Work out the finished part from the listing and answer in its coordinate system (mm). Round coordinates to 2 decimals unless told otherwise and drop trailing zeros. Loops run counter-clockwise (first coordinate to the right, second up) from the corner with the lowest first, then second, coordinate; pieces in that order, holes last.
Autodesk Inventor part; units mm, degrees
ref_plane "Work Plane1" through (0, 58, 0) normal (-1, 0, 0) x (0, 0, 1)
ref_plane "Work Plane2" through (-125, 58, 18) normal (1, 0, 0) x (0, 0, -1)
ref_plane "YZ Plane" through (0, 0, 0) normal (1, 0, 0) x (0, 1, 0)
sketch "Sketch1" plane through (0, 0, 0) normal (0, 0, 1) x (1, 0, 0)
  line L0 (-375, 40) -> (375, 40)
  line L1 (375, 40) -> (375, -40)
  line L2 (375, -40) -> (-375, -40)
  line L3 (-375, -40) -> (-375, 40)
  point P0 (0, 0)
  point P1 (375, 0)
  point P2 (0, 40)
  dimension "d0" = 750
  dimension "d1" = 80
extrude "Extrusion1" add sketch "Sketch1" along normal blind 18
sketch "Sketch2" plane through (0, 0, 18) normal (0, 0, 1) x (1, 0, 0)
  line L0 (375, 40) -> (-375, 40)
  line L1 (-375, 40) -> (-375, -40)
  line L2 (-375, -40) -> (375, -40)
  line L3 (375, -40) -> (375, 40)
  line L4 (-375, 58) -> (-316, 58)
  line L5 (-316, 58) -> (-316, 40)
  line L6 (-316, 40) -> (-375, 40)
  line L7 (-375, 40) -> (-375, 58)
  point P0 (0, 0)
  point P1 (-345.5, 40)
  point P2 (0, 40)
  point P3 (-375, 49)
  point P4 (-375, 0)
  dimension "d4" = 18
  dimension "d5" = 59
extrude "Extrusion2" add sketch "Sketch2" against normal blind 18 contours L0 L7 L4 L5
sketch "Sketch3" plane through (0, 0, 18) normal (0, 0, 1) x (1, 0, 0)
  line L0 (-175, 58) -> (-75, 58)
  line L1 (-75, 58) -> (-75, 40)
  line L2 (-75, 40) -> (-175, 40)
  line L3 (-175, 40) -> (-175, 58)
  line L4 (375, 40) -> (-316, 40)
  line L5 (-316, 58) -> (-316, 40)
  line L6 (-375, 58) -> (-316, 58)
  line L7 (-375, -40) -> (-375, 58)
  line L8 (-375, -40) -> (375, -40)
  line L9 (375, -40) -> (375, 40)
  point P0 (0, 0)
  point P1 (-125, 40)
  point P2 (29.5, 40)
  dimension "d8" = 100
  dimension "d9" = 18
  dimension "d10" = 250
extrude "Extrusion3" add sketch "Sketch3" against normal blind 18 contours L0 L1 L2 L3
sketch "Sketch4" plane through (0, 0, 18) normal (0, 0, 1) x (1, 0, 0)
  line L0 (375, 40) -> (-75, 40)
  line L1 (-75, 58) -> (-75, 40)
  line L2 (-175, 58) -> (-75, 58)
  line L3 (-175, 40) -> (-175, 58)
  line L4 (-175, 40) -> (-316, 40)
  line L5 (-316, 58) -> (-316, 40)
  line L6 (-375, 58) -> (-316, 58)
  line L7 (-375, -40) -> (-375, 58)
  line L8 (-375, -40) -> (375, -40)
  line L9 (375, -40) -> (375, 40)
  line L10 (-375, -40) -> (-357, -40)
  line L11 (-357, -40) -> (-357, 9)
  line L12 (-357, 9) -> (-375, 9)
  line L13 (-375, 9) -> (-375, -40)
  point P0 (0, 0)
  point P1 (-366, -40)
  point P2 (0, -40)
  point P3 (-375, -15.5)
  point P4 (-375, 9)
  dimension "d13" = 18
  dimension "d14" = 49
extrude "Extrusion4" cut sketch "Sketch4" against normal blind 18 contours L8 L7 L12 L11
sketch "Sketch5" plane through (0, 0, 18) normal (0, 0, 1) x (1, 0, 0)
  line L0 (-134, 58) -> (-116, 58)
  line L1 (-116, 58) -> (-116, 9)
  line L2 (-116, 9) -> (-134, 9)
  line L3 (-134, 9) -> (-134, 58)
  line L4 (-375, 9) -> (-357, 9)
  line L5 (-357, 9) -> (-357, -40)
  line L6 (-357, -40) -> (375, -40)
  line L7 (375, -40) -> (375, 40)
  line L8 (375, 40) -> (-75, 40)
  line L9 (-75, 58) -> (-75, 40)
  line L10 (-175, 58) -> (-75, 58)
  line L11 (-175, 40) -> (-175, 58)
  line L12 (-175, 40) -> (-316, 40)
  line L13 (-316, 58) -> (-316, 40)
  line L14 (-375, 58) -> (-316, 58)
  line L15 (-375, 9) -> (-375, 58)
  line L16 (-175, 58) -> (-75, 58)
  point P0 (0, 0)
  point P1 (-125, 58)
  point P2 (-125, 58)
  point P3 (-125, 58)
  dimension "d17" = 18
  dimension "d18" = 49
extrude "Extrusion5" cut sketch "Sketch5" against normal blind 18 contours L0 L1 L2 L3
ref_plane "Work Plane1" through (0, 58, 0) normal (-1, 0, 0) x (0, 0, 1)
mirror "Mirror1" about plane through (0, 58, 0) normal (-1, 0, 0) of "Extrusion5", "Extrusion4", "Extrusion3", "Extrusion2"
sketch "Sketch6" plane through (0, 0, 18) normal (0, 0, 1) x (1, 0, 0)
  line L0 (357, 9) -> (375, 9)
  line L1 (375, 9) -> (375, 58)
  line L2 (375, 58) -> (316, 58)
  line L3 (316, 58) -> (316, 40)
  line L4 (316, 40) -> (175, 40)
  line L5 (175, 40) -> (175, 58)
  line L6 (175, 58) -> (134, 58)
  line L7 (134, 58) -> (134, 9)
  line L8 (134, 9) -> (116, 9)
  line L9 (116, 9) -> (116, 58)
  line L10 (116, 58) -> (75, 58)
  line L11 (75, 58) -> (75, 40)
  line L12 (75, 40) -> (-75, 40)
  line L13 (-75, 58) -> (-75, 40)
  line L14 (-116, 58) -> (-75, 58)
  line L15 (-116, 58) -> (-116, 9)
  line L16 (-116, 9) -> (-134, 9)
  line L17 (-134, 9) -> (-134, 58)
  line L18 (-175, 58) -> (-134, 58)
  line L19 (-175, 40) -> (-175, 58)
  line L20 (-175, 40) -> (-316, 40)
  line L21 (-316, 58) -> (-316, 40)
  line L22 (-375, 58) -> (-316, 58)
  line L23 (-375, 9) -> (-375, 58)
  line L24 (-375, 9) -> (-357, 9)
  line L25 (-357, 9) -> (-357, -40)
  line L26 (-357, -40) -> (357, -40)
  line L27 (357, -40) -> (357, 9)
  point P0 (0, 0)
  point P1 (-357, 5.825)
  point P2 (-312.825, 40)
  dimension "d21" = 3.175
  dimension "d22" = 3.175
hole "Hole1" at (-357, 5.825, 18) at (-312.825, 40, 18) direction (0, 0, -1) diameter 6.35 end through all
mirror "Mirror2" about plane through (0, 58, 0) normal (-1, 0, 0) of "Hole1"
sketch "Sketch7" plane through (0, 0, 18) normal (0, 0, 1) x (1, 0, 0)
  arc A0 (357, 9) -> (357, 2.65) centre (357, 5.825) ccw
  line L0 (357, 9) -> (375, 9)
  line L1 (375, 9) -> (375, 58)
  line L2 (375, 58) -> (316, 58)
  line L3 (316, 58) -> (316, 40)
  arc A1 (309.65, 40) -> (316, 40) centre (312.825, 40) ccw
  line L4 (309.65, 40) -> (175, 40)
  line L5 (175, 40) -> (175, 58)
  line L6 (175, 58) -> (134, 58)
  line L7 (134, 58) -> (134, 9)
  line L8 (134, 9) -> (116, 9)
  line L9 (116, 9) -> (116, 58)
  line L10 (116, 58) -> (75, 58)
  line L11 (75, 58) -> (75, 40)
  line L12 (75, 40) -> (-75, 40)
  line L13 (-75, 58) -> (-75, 40)
  line L14 (-116, 58) -> (-75, 58)
  line L15 (-116, 58) -> (-116, 9)
  line L16 (-116, 9) -> (-134, 9)
  line L17 (-134, 9) -> (-134, 58)
  line L18 (-175, 58) -> (-134, 58)
  line L19 (-175, 40) -> (-175, 58)
  line L20 (-175, 40) -> (-309.65, 40)
  arc A2 (-316, 40) -> (-309.65, 40) centre (-312.825, 40) ccw
  line L21 (-316, 58) -> (-316, 40)
  line L22 (-375, 58) -> (-316, 58)
  line L23 (-375, 9) -> (-375, 58)
  line L24 (-375, 9) -> (-357, 9)
  arc A3 (-357, 2.65) -> (-357, 9) centre (-357, 5.825) ccw
  line L25 (-357, 2.65) -> (-357, -40)
  line L26 (-357, -40) -> (357, -40)
  line L27 (357, -40) -> (357, 2.65)
  point P0 (0, 0)
  point P1 (-178.175, 40)
  point P2 (-134, 12.175)
  point P3 (-242.325, 40)
  dimension "d30" = 3.175
  dimension "d31" = 3.175
hole "Hole2" at (-178.175, 40, 18) at (-134, 12.175, 18) direction (0, 0, -1) diameter 6.35 end through all
ref_plane "Work Plane2" through (-125, 58, 18) normal (1, 0, 0) x (0, 0, -1)
mirror "Mirror3" about plane through (-125, 58, 18) normal (1, 0, 0) of "Hole2"
mirror "Mirror4" about plane through (0, 58, 0) normal (-1, 0, 0) of "Hole2", "Mirror3"
equation "\"d0\" = tableWidth"
equation "\"d1\" = legTopDepth"
equation "\"d2\" = plyThickness"
equation "\"d4\" = legTopTabHeight"
equation "\"d5\" = 0.5 * plyThickness + 0.5 * legTabTotalWidth"
equation "\"d6\" = plyThickness"
equation "\"d8\" = legTabTotalWidth"
equation "\"d9\" = legTopTabHeight"
equation "\"d11\" = plyThickness"
equation "\"d13\" = plyThickness"
equation "\"d14\" = legTopSlotDepth"
equation "\"d15\" = plyThickness"
equation "\"d17\" = plyThickness"
equation "\"d18\" = legTopSlotDepth"
equation "\"d19\" = plyThickness"
equation "\"d23\" = millDiameter"
equation "\"d32\" = millDiameter"
equation "\"plyThickness\" = 18"
equation "\"legHeight\" = 702"
equation "\"tableWidth\" = 750"
equation "\"legTopDepth\" = 80"
equation "\"millDiameter\" = 6.35"
equation "\"legTopTabHeight\" = 18"
equation "\"legTabTotalWidth\" = 100"
equation "\"legTopSlotDepth\" = 49"
properties part number "shortSlat"
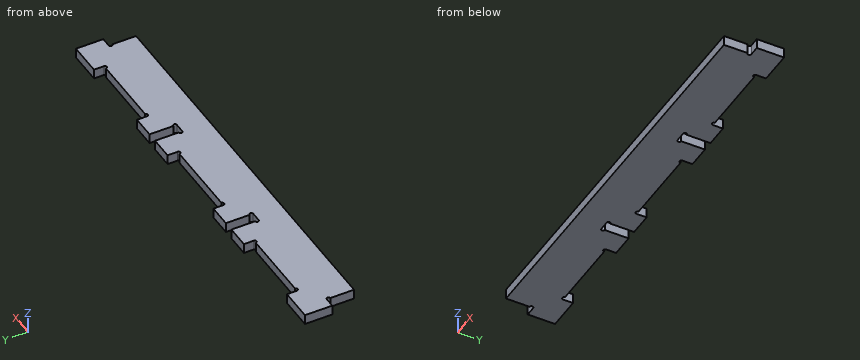
Item 1: Section B-B, the plane x = 35 is taken. Give the vertices of the cut face in (y, z).
Item 2: Each of these flat-tipped pins is pushed along its axis until it touches: P1, Ø9, axis at x = -126.5, z = 6, coming from the +Y side; P2, Ø3, axis at y = -22.5, z = 13, coming from the -X side; P3, Ø9, axis at x = -363, z = 7, coming from the -Y side. Where does it stop, or does it pass through?
Item 3: Section A-A, the plane y = 30.5 is taken. Give the vertices of the cut face in (x, z), plus the area to 3 significant figures.
Item 4: Straight lines are drawn through the part: line 1 (X direction, y = 43.5, z = 17); line 2 (X direction, y = 23.5, z = 11); line 3 (X direction, y = 11, z = 12.75). For each, find the intervals that lie inside material, in ascending order.
Answer below:
1. outline: (-40, 0) - (40, 0) - (40, 18) - (-40, 18) - close
2. P1: stops at y = 9
2. P2: stops at x = -357
2. P3: stops at y = 9
3. outline: (-375, 0) - (-134, 0) - (-134, 18) - (-375, 18) - close; (-116, 0) - (116, 0) - (116, 18) - (-116, 18) - close; (134, 0) - (375, 0) - (375, 18) - (134, 18) - close
3. area: 12,900 mm2
4. line 1: x = -375 to -316, -175 to -134, -116 to -75, 75 to 116, 134 to 175, 316 to 375
4. line 2: x = -375 to -134, -116 to 116, 134 to 375
4. line 3: x = -375 to -136.95, -113.05 to 113.05, 136.95 to 375
